```python
from build123d import *

# Parameters (mm, degrees)
SKETCH1_R                 = 39
BOSS_EXTRUDE1_DEPTH       = 98
SKETCH2_R                 = 4.7625
BOSS_EXTRUDE2_DEPTH       = 14.2875
M6X1_0_TAPPED_HOLE1_D     = 5
M6X1_0_TAPPED_HOLE1_DEPTH = 14.9987
M6X1_0_TAPPED_HOLE1_TIP   = 1.502151548


with BuildPart() as part:
    # Sketch1 → Boss-Extrude1 (new body)
    with BuildSketch(Plane.XY):
        Circle(SKETCH1_R)
    extrude(amount=BOSS_EXTRUDE1_DEPTH)

    # Sketch2 → Boss-Extrude2 (add)
    with BuildSketch(Plane.XY.offset(98)):
        Circle(SKETCH2_R)
    extrude(amount=BOSS_EXTRUDE2_DEPTH)

    # M6x1.0 Tapped Hole1
    with Locations(Plane.XY.offset(98)):
        with Locations((0, 17.5), (15.155444566, -8.75), (-15.155444566, -8.75)):
            Hole(M6X1_0_TAPPED_HOLE1_D / 2, depth=M6X1_0_TAPPED_HOLE1_DEPTH)
            with Locations((0, 0, -(M6X1_0_TAPPED_HOLE1_DEPTH + M6X1_0_TAPPED_HOLE1_TIP / 2))):  # 118° drill point
                Cone(0, M6X1_0_TAPPED_HOLE1_D / 2, M6X1_0_TAPPED_HOLE1_TIP, mode=Mode.SUBTRACT)


solid = part.part
```
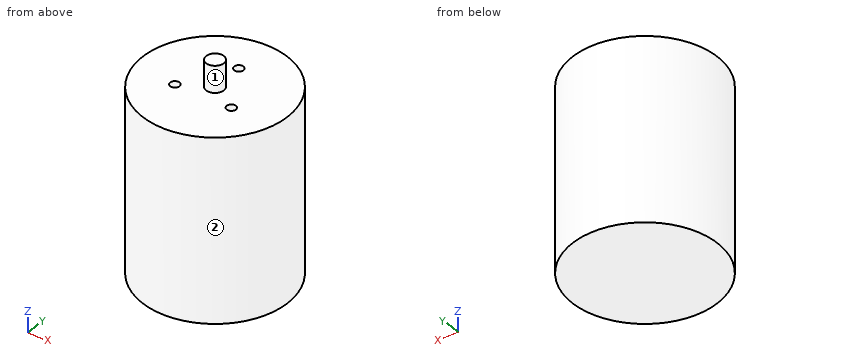
Geometry check sheet. Reference: the model listing, model coordinates, mm. Face numbers are marked on the shaded views. A direction names the side the tool comes from. Round coordinates to 2 decimals unless told otherwise and drop trailing zeros. Loops run counter-clockwise (first coordinate to the right, second up) from the corner with the lowest first, then second, coordinate; pieces in that order, holes last. Notation, with made-up numbers: (-18, 17.25) - (24, 17.25) arc R28 cw to (24, 47.25) - close; hole circle Ø10 at (57, 51.25). An arc over 180 degrees is marked (long way). Use a Markdown table: item, result.
Q1. Cross-section at B-B on z = 65.5. Record the cut outline in (x, y), plus the area to 3 significant figures.
Solutions:
| item | result |
|---|---|
| outline | circle Ø78 at (0, 0) |
| area | 4,780 mm2 |
Q2. Cross-section at C-C on x = -30.5. Record the cut outline in (y, z).
Solutions:
| item | result |
|---|---|
| outline | (-24.31, 0) - (24.31, 0) - (24.31, 98) - (-24.31, 98) - close |
Q3. Cross-section at A-A on y = 0. Record the cut outline in (x, z), plus the area to 3 significant figures.
Solutions:
| item | result |
|---|---|
| outline | (-39, 0) - (39, 0) - (39, 98) - (4.76, 98) - (4.76, 112.29) - (-4.76, 112.29) - (-4.76, 98) - (-39, 98) - close |
| area | 7,780 mm2 |
Q4. Material ranges on line 1 (X direction, y = -8, z = 87); line 2 (Y direction, x = 0.5, z = 10); line 3 (Z direction, x = 35, y = 4), recorded low to high.
Solutions:
| item | result |
|---|---|
| line 1 | x = -38.17 to -17.54, -12.77 to 12.77, 17.54 to 38.17 |
| line 2 | y = -39 to 39 |
| line 3 | z = 0 to 98 |
Q5. Access from +Z, -Z, +X, -X, +Y, -Y to the whole of each face (thin tool, end or side, straight path). Record for the marked faces 1 and 2.
Solutions:
| item | result |
|---|---|
| face 1 | +Z |
| face 2 | +Z, -Z |
Q6. Go/stop test with flat-tipped pins: P1, Ø1.5, axis at y = 18, z = 28.5, coming from the -X side; P2, Ø4, axis at x = -15.16, y = -8.75, coming from the +Z side; P3, Ø1, axis at x = 4, y = -31, coming from the +Z side. Record where each tip stops, or that it passes through.
Solutions:
| item | result |
|---|---|
| P1 | stops at x = -34.98 |
| P2 | stops at z = 82.7 |
| P3 | stops at z = 98 |
Q7. Cross-section at D-D on y = -28. Record the cut outline in (x, z).
Solutions:
| item | result |
|---|---|
| outline | (-27.15, 0) - (27.15, 0) - (27.15, 98) - (-27.15, 98) - close |
